Source: CAD feature listing. Evaluate the final solid. Frame: model axes, mm. A direction names the side the tool comes from. Give positions to 0.01 mm unless a question says otherwise; leave off trailing zeros. Write each loop counter-clockwise with the first axis right and the second up, starting at its lowest first coordinate (ties: lowest second). Pieces come first, ordered by that corner, then holes. Notation, with made-up numbers: M 89.5,13.5 L 144.5,13.5 A20 cw 144.5,35.5 Z; hole C 28.5,10.5 d4. An arc over 180 degrees is marked long. Answer as a JSON object with one key per item and string values. Group by question number.
```python
from build123d import *

# Parameters (mm, degrees)
F0_W     = 26.0096
F0_H     = 26.0096
F1_DEPTH = 26.0096
F2_R     = 4.795051
F3_DEPTH = 1.2
F4_DEPTH = 12


with BuildPart() as f1:
    # F0 (on Top) → F1 (new body)
    with BuildSketch(Plane.XY):
        Rectangle(F0_W, F0_H)
    extrude(amount=F1_DEPTH)

    # F2 (on Top) → F3 (join)
    with BuildSketch(Plane.XY):
        Circle(F2_R)
    extrude(amount=-F3_DEPTH)

    # F2 (on Top) → F4 (join)
    with BuildSketch(Plane.XY):
        Circle(F2_R)
    extrude(amount=-F4_DEPTH)


solid = f1.part
```
(1) Section A-A, the plane y = 0. Return loops of the section in (x, z).
(2) Ray query, L1, parallel to Z at x = 8, y = -1.5; L2, parallel to X at y = 0.25, z = -2; L3, parallel to X at y = 1.25, z = -9.5. Return the intervals inside material, ascending. Write a range as [from, to].
(3) Section C-C, the plane x = -7.75. Return loops of the section in (y, z).
(4) Access query for faces 1 (the cylindrical face through (-1.04, -4.68, -5.92)), 2 (the flat face through (0, -13.005, 13)). Directions: +Z, -Z, +X, -X, +Y, -Y. A direction counts if a zero-diameter tool reaches every point of the face in a straight line with its end or side. Return the directions, or none.
Reported:
{
 "1": {"outline": "M -13,0 L -4.8,0 L -4.8,-12 L 4.8,-12 L 4.8,0 L 13,0 L 13,26.01 L -13,26.01 Z"},
 "2": {"L1": "z = [0, 26.01]", "L2": "x = [-4.79, 4.79]", "L3": "x = [-4.63, 4.63]"},
 "3": {"outline": "M -13,0 L 13,0 L 13,26.01 L -13,26.01 Z"},
 "4": {"face 1": "-Z", "face 2": "+Z, -Z, +X, -X, -Y"}
}
